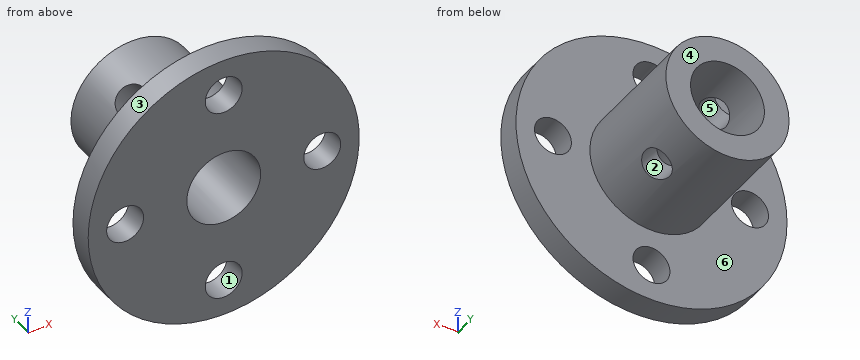
Autodesk Inventor part; units mm, degrees
ref_plane "YZ Plane" through (0, 0, 0) normal (1, 0, 0) x (0, 1, 0)
ref_plane "XZ Plane" through (0, 0, 0) normal (0, 1, 0) x (-1, 0, 0)
ref_plane "XY Plane" through (0, 0, 0) normal (0, 0, 1) x (1, 0, 0)
sketch "Schizzo1" plane through (0, 0, 0) normal (0, 1, 0) x (-1, 0, 0)
  circle A0 centre (0, 0) radius 11
  dimension "d0" = 22
extrude "Estrusione1" add sketch "Schizzo1" along normal blind 2
sketch "Schizzo2" plane through (0, 2, 0) normal (0, 1, 0) x (1, 0, 0)
  circle A0 centre (0, 0) radius 5
  line L0 (-7, -1) -> (-1, 7)
  line L1 (-1, 7) -> (7, 1)
  line L2 (7, 1) -> (1, -7)
  line L3 (1, -7) -> (-7, -1)
  point P0 (-3, -4)
  point P1 (4, -3)
  point P2 (-4, 3)
  point P3 (3, 4)
  dimension "d3" = 10
extrude "Estrusione2" add sketch "Schizzo2" along normal blind 10
sketch "Schizzo3" plane through (0, 0, 0) normal (0, -1, 0) x (1, 0, 0)
  circle A0 centre (0, 0) radius 2
  circle A1 centre (-8, 0) radius 1.5
  line L0 (0, -8) -> (0, 8)
  line L1 (-8, 0) -> (8, 0)
  circle A2 centre (0, -8) radius 1.5
  circle A3 centre (8, 0) radius 1.5
  circle A4 centre (0, 8) radius 1.5
  dimension "d6" = 4
  dimension "d7" = 3
  dimension "d8" = 16
  dimension "d9" = 16
  dimension "d10" = 3
  dimension "d11" = 3
  dimension "d12" = 3
extrude "Estrusione3" cut sketch "Schizzo3" against normal blind 2 contours A2 | A1 | A4 | A3
sketch "Schizzo4" plane through (0, 0, 0) normal (0, -1, 0) x (1, 0, 0)
  circle A0 centre (0, 0) radius 3
  dimension "d15" = 6
extrude "Estrusione4" cut sketch "Schizzo4" against normal blind 12
sketch "Schizzo5" plane through (1, 2, 7) normal (-0.6, 0, 0.8) x (0.8, 0, 0.6)
  line L0 (-0.7385, 0) -> (-9.9134, 0)
  line L1 (-5, 0) -> (-5, 4)
  line L2 (-5, 0) -> (-1, 0) construction
  line L3 (-5, 4) -> (-5, 5.5)
  point P0 (-5, -2)
  dimension "d19" = 4
  dimension "d20" = 90
  dimension "d21" = 1.5
  dimension "d22" = 180
hole "Foro1" at (-3, 7.5, 4) direction (0.6, 0, -0.8) diameter 2.459 depth 6 tip angle 118
sketch "Schizzo7" plane through (-1, 2, -7) normal (0.6, 0, -0.8) x (-0.8, 0, -0.6)
  circle A0 centre (-5, 5.5) radius 1.2295
  circle A1 centre (-5, 5.5) radius 1.2295
  point P0 (-5, -2)
  point P1 (-6.2295, 5.5)
hole "Foro2" at (3, 7.5, -4) direction (-0.6, 0, 0.8) diameter 2.459 depth 6 tip angle 118
sketch "Schizzo6" plane through (0, 12, 0) normal (0, 1, 0) x (1, 0, 0)
  circle A0 centre (0, 0) radius 5
  circle A1 centre (0, 0) radius 3
  line L0 (-1, 7) -> (-7, -1)
  line L1 (-1, 7) -> (7, 1)
  line L2 (7, 1) -> (1, -7)
  line L3 (1, -7) -> (-7, -1)
  line L4 (-7, -1) -> (-1, 7)
  point P0 (-4, 3)
  point P1 (-3, -4)
  point P2 (4, -3)
  point P3 (-4, 3)
  point P4 (3, 4)
extrude "Estrusione5" cut sketch "Schizzo6" against normal blind 10 contours A0 L1 L2 | A0 L0 L1 | L2 L3 A0 | A0 L3 L0
properties part number "9_Flangia" material "Acciaio, Dolce"
Input: part model. Units: mm. Frame: model coordinates. Face numbers are marked on the shaded views. A direction names the side the tool comes from. Coordinates: 2 decimals unless noted, no trailing zeros. Loops run counter-clockwise (first coordinate to the right, second up) from the corner with the lowest first, then second, coordinate; pieces in that order, holes last.
Q1. Cut plane C-C (x = 8). Output: boundary loops of the cut face in (y, z), then the cut area to 3 significant figures.
Q2. Material intervals for line 1 (Z direction, x = 0, y = 1.15); line 2 (Z direction, x = 0, y = 7.5); line 3 (Y direction, x = 4, z = -5.75), sorted ascending.
Q3. Set-up query: the marked faces 5 and 6. Return all of +Z, -Z, +X, -X, +Y, -Y with unobstructed straight access to the full face (end or side cutting, diameter ignored); none if empty.
Q4. Contact query for flat-ended pins moving along their axis: pin 1 (2.5 mm diameter, centred on x = 0, z = 8, fed in from -Y); pin 2 (5 mm diameter, centred on x = 1, y = 7, fed in from -Z); pin 3 (1.5 mm diameter, centred on y = 2, z = 8, fed in from -X). Output: stop coordinate, or through.
Q5. Cut plane B-B (z = 7.5). Output: boundary loops of the cut face in (x, y), then the cut area to 3 significant figures.
Q6. Draft query along Z for the marked faces 1, 2, 3 and 4. Return one class per face: +Z half, -Z half, draft (parallel to the pull), parting line (faces both ways), or undercut.
Q7. Cut plane D-D (y = 6). Output: boundary loops of the cut face in (x, z).
Q8. Cut plane A-A (x = 0). Output: boundary loops of the cut face in (y, z), then the cut area to 3 significant figures.
Working result:
1. outline: (0, -7.55) - (2, -7.55) - (2, -1.5) - (0, -1.5) - close; (0, 1.5) - (2, 1.5) - (2, 7.55) - (0, 7.55) - close
1. area: 24.2 mm2
2. line 1: z = -11 to -9.5, -6.5 to -3, 3 to 6.5, 9.5 to 11
2. line 2: z = -5 to -3, 3 to 5
2. line 3: y = 0 to 2
3. face 5: none
3. face 6: +Y
4. pin 1: passes through
4. pin 2: stops at z = -5
4. pin 3: stops at x = -8.27
5. outline: (-8.05, 0) - (-1.41, 0) - (-1.41, 2) - (-8.05, 2) - close; (1.41, 0) - (8.05, 0) - (8.05, 2) - (1.41, 2) - close
5. area: 26.5 mm2
6. face 1: undercut
6. face 2: undercut
6. face 3: parting line
6. face 4: draft
7. outline: circle Ø10 at (0, 0); hole circle Ø6 at (0, 0)
8. outline: (0, -11) - (2, -11) - (2, -9.5) - (0, -9.5) - close; (0, -6.5) - (2, -6.5) - (2, -5) - (12, -5) - (12, -3) - (0, -3) - close; (0, 3) - (12, 3) - (12, 5) - (2, 5) - (2, 6.5) - (0, 6.5) - close; (0, 9.5) - (2, 9.5) - (2, 11) - (0, 11) - close
8. area: 60.0 mm2
